Autodesk Inventor part; units mm, degrees
ref_plane "Work Plane1" through (0, -14.4489, 10.16) normal (1, 0, 0) x (0, 0, -1)
ref_plane "YZ Plane" through (0, 0, 0) normal (1, 0, 0) x (0, 1, 0)
ref_plane "XZ Plane" through (0, 0, 0) normal (0, 1, 0) x (-1, 0, 0)
sketch "Sketch1" plane through (0, 0, 0) normal (0, 0, 1) x (1, 0, 0)
  circle A0 centre (0, 0) radius 20.32
  dimension "d0" = 40.64
extrude "Extrusion1" add sketch "Sketch1" along normal blind 10.16
sketch "Sketch2" plane through (0, 0, 10.16) normal (0, 0, 1) x (1, 0, 0)
  point P0 (0, 0)
  point P1 (0, 0)
hole "Hole1" at (0, 0, 10.16) direction (0, 0, -1) diameter 9.652 depth 10.9728 tip angle 118
sketch "Sketch3" plane through (0, 0, 10.16) normal (0, 0, 1) x (1, 0, 0)
  point P0 (0, 0)
  point P1 (0, 14.2875)
  point P2 (0, -14.2875)
  dimension "d10" = 28.575
  dimension "d11" = 14.2875
hole "Hole2" at (0, 14.2875, 10.16) at (0, -14.2875, 10.16) direction (0, 0, -1) diameter 6.604 depth 10.9728 tip angle 118
sketch "Sketch4" plane through (0, 0, 10.16) normal (0, 0, 1) x (1, 0, 0)
  line L0 (-14.2875, -38.2443) -> (14.2875, -38.2443)
  line L1 (14.2875, -38.2443) -> (14.2875, 37.8114)
  line L2 (14.2875, 37.8114) -> (-14.2875, 37.8114)
  line L3 (-14.2875, 37.8114) -> (-14.2875, -38.2443)
  line L4 (-54.4025, 52.7865) -> (43.8573, 52.7865)
  line L5 (43.8573, 52.7865) -> (43.8573, -66.4941)
  line L6 (43.8573, -66.4941) -> (-54.4025, -66.4941)
  line L7 (-54.4025, -66.4941) -> (-54.4025, 52.7865)
  point P0 (0, 0)
  dimension "d19" = 28.575
  dimension "d20" = 14.2875
extrude "Extrusion2" cut sketch "Sketch4" against normal blind 10.16
sketch "Sketch5" plane through (-14.2875, -14.4489, 10.16) normal (-1, 0, 0) x (0, 0, 1)
  line L0 (0, 0) -> (-10.16, 0)
  line L1 (0, 28.8977) -> (0, 0)
  line L2 (-10.16, 28.8977) -> (0, 28.8977)
  line L3 (-10.16, 0) -> (-10.16, 28.8977)
  point P0 (-10.16, 14.4489)
  point P1 (-5.08, 23.9739)
  point P2 (-5.08, 4.9239)
  dimension "d23" = 10.16
  dimension "d24" = 5.08
  dimension "d25" = 5.08
  dimension "d26" = 19.05
  dimension "d27" = 28.8977
  dimension "d28" = 4.9239
hole "Hole3" at (-14.2875, 9.525, 5.08) at (-14.2875, -9.525, 5.08) direction (1, 0, 0) diameter 5.08 depth 10.9728 tip angle 118
ref_plane "Work Plane1" through (0, -14.4489, 10.16) normal (1, 0, 0) x (0, 0, -1)
mirror "Mirror1" about plane through (0, -14.4489, 10.16) normal (1, 0, 0) of "Hole3"
Verification items for the finished model (mm, model axes). A direction names the side the tool comes from. Round coordinates to 2 decimals unless told otherwise and drop trailing zeros. Write each loop counter-clockwise with the first axis right and the second up, starting at its lowest first coordinate (ties: lowest second). Pieces come first, ordered by that corner, then holes.
1. Access from +Z, -Z, +X, -X, +Y, -Y to the whole of each face (thin tool, end or side, straight path). Record for faces 4 (the cylindrical face through (8.724, 7.045, 4.529)), 5 (the cylindrical face through (0.22, -20.32, 5.01)), 6 (the cylindrical face through (-8.724, -7.045, 4.529)).
2. Scan lines: L1, parallel to Y at x = 9.25, z = 5.08 (3 decimals); L2, parallel to Y at x = 6.5, z = 5.08 (3 decimals); L3, parallel to Z at x = -11.5, y = 9.5. Record each from-to range of solid material in increasing order.
3. Section check A-A on x = 0. Enter the section's corners in (y, z).
4. Section check B-B on y = 0. Enter the section's corners in (x, z).
5. Draft check along Z on faces 1 (the flat face through (-3, -4, 10.16)), 2 (the cylindrical face through (8.724, -11.071, 3.064)), 3 (the cylindrical face through (2.937, 3.83, 5.009)). Enter one of: +Z half, -Z half, draft (parallel to the pull), parting line (faces both ways), or undercut.
6. Gauge pin test, flat ends, axial feed: P1, Ø4, axis at x = 1, y = 0.5, coming from the +Z side; P2, Ø1, axis at x = 5.5, y = 1, coming from the -Z side; P3, Ø4, axis at x = 7.5, z = 9, coming from the -Y side. Record the tip position at first contact, or that the pin passes through.
7. Section check D-D on z = 7. State how many separate pieces and enclosed holes the cut face has, plus the area to 3 significant figures.
8. Section check C-C on x = -8. Enter the section's corners in (y, z) (3 decimals), plus the area to 3 significant figures.
Answer:
1. face 4: +X
1. face 5: +Z, -Z, -Y
1. face 6: -X
2. L1: y = -18.093 to -12.065, -6.985 to 6.985, 12.065 to 18.093
2. L2: y = -19.252 to -12.065, -6.985 to 6.985, 12.065 to 19.252
2. L3: z = 0 to 2.54, 7.62 to 10.16
3. outline: (-20.32, 0) - (-17.59, 0) - (-17.59, 10.16) - (-20.32, 10.16) - close; (-10.99, 0) - (-4.83, 0) - (-4.83, 10.16) - (-10.99, 10.16) - close; (4.83, 0) - (10.99, 0) - (10.99, 10.16) - (4.83, 10.16) - close; (17.59, 0) - (20.32, 0) - (20.32, 10.16) - (17.59, 10.16) - close
4. outline: (-14.29, 0) - (-4.83, 0) - (-4.83, 10.16) - (-14.29, 10.16) - close; (4.83, 0) - (14.29, 0) - (14.29, 10.16) - (4.83, 10.16) - close
5. face 1: +Z half
5. face 2: undercut
5. face 3: draft
6. P1: passes through
6. P2: stops at z = 0
6. P3: stops at y = -19.56
7. separate pieces: 1
7. enclosed holes: 3
7. area: 766 mm2
8. outline: (-18.679, 0) - (18.679, 0) - (18.679, 10.16) - (-18.679, 10.16) - close; hole circle Ø5.08 at (-9.525, 5.08); hole circle Ø5.08 at (9.525, 5.08)
8. area: 339 mm2
